from build123d import *

# Parameters (mm, degrees)
F1_DEPTH   = 95
F3_DEPTH   = 10.001
F4_W       = 59
F4_H       = 24
F1_FACE2_W = 95
F1_FACE2_H = 52.2015325446
F5_DEPTH   = 56.001


with BuildPart() as f1:
    # F0 (on Right) → F1 (new body)
    with BuildSketch(Plane.YZ):
        Polygon((-60, 0), (0, 0), (0, 56), (-10, 56), (-10, 28), (-60, 13), align=None)
    extrude(amount=F1_DEPTH)

    # F2 (on face) → F3 (cut, through all)
    with BuildSketch(Plane.XZ.offset(10)):
        Polygon((95, 56), (56, 56), (95, 28), align=None)
    extrude(amount=-F3_DEPTH, mode=Mode.SUBTRACT)

    # F4 (on face) + F1_face2 (on face) → F5 (cut, through all)
    with BuildSketch(Plane(origin=(0, 0, 0), x_dir=(1, 0, 0), z_dir=(0, 0, -1))):
        with Locations((48.5, 48)):
            Rectangle(F4_W, F4_H)
    with BuildSketch(Plane(origin=(47.5, -35, 20.5), x_dir=(1, 0, 0), z_dir=(0, -0.2873478856, 0.9578262852))):
        Rectangle(F1_FACE2_W, F1_FACE2_H)
    extrude(amount=-F5_DEPTH, dir=(0, 0, -1), mode=Mode.SUBTRACT)


solid = f1.part
CAD build for the part. Positions are in the model's coordinates, mm. A direction names the side the tool comes from. Round coordinates to 2 decimals unless told otherwise and drop trailing zeros. Loops run counter-clockwise (first coordinate to the right, second up) from the corner with the lowest first, then second, coordinate; pieces in that order, holes last.
(1) Two-plate mould, pull along X, no slides. Class faces 1 (the flat face through (95, -24, 11)), 2 (the flat face through (0, -24, 16)), 3 (the flat face through (48, -36, 10)), 4 (the flat face through (47, -24, 0)): +X half, -X half, draft (parallel to the pull), parting line (faces both ways), or undercut.
(2) Drop flat-ended pins along their axis: pin 1 (8.5 mm diameter, centred on x = 69.5, z = 39.5, fed in from -Y); pin 2 (16 mm diameter, centred on x = 62, z = 14.5, fed in from -Y). Give the stop position or say it passes through.
(3) Cut at B-B (x = 35). Give the cut face in (y, z), plus the area to 3 significant figures.
(4) Which spindle directions (+Z, -Z, +X, -X, +Y, -Y) get a long thin tool onto all of the face, cutting with end or side? Do faces 5 (the flat face through (19, -48, 8)), 6 (the flat face through (47, 0, 28)), 7 (the flat face through (36, -10, 42)). Say none if no direction does.
(5) Cut at A-A (y = -38.5). Give the cut face in (x, z), plus the area to 3 significant figures.
(6) Cut at D-D (z = 25). Give the cut face in (x, y).
(7) Cut at C-C (y = -7). Give the cut face in (x, z).
(8) Wall check: line 1 along X through (y, z) = (-55, 8); line 2 along Y through (x, z) = (15, 48); line 3 along Y through (x, z) = (41.5, 13.5). Give the ranges that are in metal, low to high.
Findings below:
1. face 1: +X half
1. face 2: -X half
1. face 3: undercut
1. face 4: draft
2. pin 1: stops at y = -10
2. pin 2: stops at y = -36
3. outline: (-36, 0) - (0, 0) - (0, 56) - (-10, 56) - (-10, 28) - (-36, 20.2) - close
3. area: 1,190 mm2
4. face 5: +Z, -Z, -Y
4. face 6: +Z, -Z, +X, -X, +Y
4. face 7: +Z, +X, -X, -Y
5. outline: (0, 0) - (19, 0) - (19, 19.45) - (0, 19.45) - close; (78, 0) - (95, 0) - (95, 19.45) - (78, 19.45) - close
5. area: 700 mm2
6. outline: (0, -20) - (95, -20) - (95, 0) - (0, 0) - close
7. outline: (0, 0) - (95, 0) - (95, 28) - (56, 56) - (0, 56) - close
8. line 1: x = 0 to 19, 78 to 95
8. line 2: y = -10 to 0
8. line 3: y = -36 to 0
